```python
from build123d import *

# Parameters (mm, degrees)
F1_DEPTH = 2


with BuildPart() as f1:
    # F0 (on Top) → F1 (new body)
    with BuildSketch(Plane.XY):
        with BuildLine():
            Line((4.733724, -4.386716), (4.733724, -3.120114))
            ThreePointArc((4.733724, -3.120114), (0.208889, 1.143126), (-4.315945, -3.120114))
            Line((-4.315945, -3.120114), (-4.315945, -4.386716))
            Line((-4.315945, -4.386716), (4.733724, -4.386716))
        make_face()
        with BuildLine():
            ThreePointArc((-4.14372, -3.151427), (0.201964, 0.973099), (4.577155, -3.120114))
            Line((4.577155, -3.120114), (3.955484, -3.151427))
            Line((3.955484, -3.151427), (3.568369, -3.014677))
            Line((3.568369, -3.014677), (1.677037, -0.935318))
            Line((1.677037, -0.935318), (1.190378, -0.603505))
            Line((1.190378, -0.603505), (0.371907, 0.336631))
            Line((0.371907, 0.336631), (0.679859, -0.437599))
            Line((0.679859, -0.437599), (0.847505, -0.603505))
            Line((0.847505, -0.603505), (1.079774, -0.935318))
            Line((1.079774, -0.935318), (1.787641, -1.51046))
            Line((1.787641, -1.51046), (2.030971, -1.897575))
            Line((2.030971, -1.897575), (3.170194, -3.014677))
            Line((3.170194, -3.014677), (3.170194, -3.151427))
            Line((3.170194, -3.151427), (2.030971, -3.151427))
            Line((2.030971, -3.151427), (1.677037, -2.328931))
            Line((1.677037, -2.328931), (1.190378, -1.51046))
            Line((1.190378, -1.51046), (0.679859, -1.03181))
            Line((0.679859, -1.03181), (0.604176, -0.761511))
            Line((0.604176, -0.761511), (0.468727, -0.277765))
            Line((0.468727, -0.277765), (0.371907, -0.304874))
            Line((0.371907, -0.304874), (0.604176, -1.134406))
            Line((0.604176, -1.134406), (1.079774, -1.753789))
            Line((1.079774, -1.753789), (1.466889, -2.616502))
            Line((1.466889, -2.616502), (1.466889, -3.151427))
            Line((1.466889, -3.151427), (-0.822619, -3.151427))
            Line((-0.822619, -3.151427), (-0.822619, -3.014677))
            Line((-0.822619, -3.014677), (-0.512927, -2.793469))
            Line((-0.512927, -2.793469), (0.217061, -1.610004))
            Line((0.217061, -1.610004), (0, 0.458295))
            Line((0, 0.458295), (-0.822619, -0.304874))
            Line((-0.822619, -0.304874), (-1.618969, -1.388795))
            Line((-1.618969, -1.388795), (-1.818057, -1.388795))
            Line((-1.818057, -1.388795), (-3.233791, -3.014677))
            Line((-3.233791, -3.014677), (-3.47712, -3.014677))
            Line((-3.47712, -3.014677), (-3.654087, -3.151427))
            Line((-3.654087, -3.151427), (-4.14372, -3.151427))
        make_face(mode=Mode.SUBTRACT)
    extrude(amount=F1_DEPTH)


solid = f1.part
```
CAD build for the part. Positions are in the model's coordinates, mm. A direction names the side the tool comes from. Coordinates: 2 decimals unless noted, no trailing zeros. Write each loop counter-clockwise with the first axis right and the second up, starting at its lowest first coordinate (ties: lowest second). Pieces come first, ordered by that corner, then holes. Notation, with made-up numbers: (14, 69) -> (53, 69) arc R21 cw to (53, 79) -> close; hole circle Ø11 at (35, 17). An arc over 180 degrees is marked (long way). Use CSV: the item, a comma, the result in double quotes. Start each with the question number.
Item 1: Two-plate mould, pull along Y, no slides. Class faces 1 (the flat face through (-1, -3, 0)), 2 (the flat face through (3, -3.151, 1)), 3 (the cylindrical face through (0.305, 1.142, 0.986)), 4 (the flat face through (1.27, -2.18, 0.99)): +Y half, -Y half, draft (parallel to the pull), parting line (faces both ways), or undercut.
Item 2: Wall check: probe 1 along Y at (x, z) = (2.5, 0.2); probe 2 along X at (y, z) = (-1.9, 0.3); probe 3 along Y at (x, z) = (3, 0.3). Give the ranges that are in metal, low to high.
Item 3: Tool access for faces 5 (the flat face through (0, -4.387, 1)), 6 (the flat face through (-0.41, 0.08, 0.99)): list every direction of +Z, -Z, +X, -X, +Y, -Y with a clear straight run to the whole face (end or side of a thin tool).
Item 4: Drop a flat-ended pin along its axis: P1, Ø0.9, axis at x = 2.5, z = 1.5, coming from the +Y side. Give the stop position or say it passes through.
Item 5: Band-saw the part on D-D, the plane y = -2.5. Write the cut outline in (x, z), plus the area to 3 significant figures.
Item 6: Band-saw the part on C-C, the plane x = 2.5. Write the cut outline in (y, z), plus the area to 3 significant figures.
Item 7: Band-saw the part on B-B, the plane y = 0.8. Write the cut outline in (x, z).
Item 8: Band-saw the part on A-A, the plane x = -2. Write the cut outline in (y, z).
Response values:
1,face 1,"draft"
1,face 2,"undercut"
1,face 3,"+Y half"
1,face 4,"undercut"
2,probe 1,"y = -4.39 to -3.15, -2.36 to -1.84, 0.33 to 0.52"
2,probe 2,"x = -4.07 to -3.89, -2.26 to 0.04, 1.15 to 1.42, 2.03 to 2.55, 4.32 to 4.49"
2,probe 3,"y = -4.39 to -3.15, -2.85 to -2.39, -0.03 to 0.18"
3,face 5,"+Z, -Z, +X, -X, -Y"
3,face 6,"+Z, -Z"
4,P1,"stops at y = 0.75"
5,outline,"(-4.24, 0) -> (-4.06, 0) -> (-4.06, 2) -> (-4.24, 2) -> close; (-2.79, 0) -> (-0.33, 0) -> (-0.33, 2) -> (-2.79, 2) -> close; (1.41, 0) -> (1.75, 0) -> (1.75, 2) -> (1.41, 2) -> close; (2.65, 0) -> (3.1, 0) -> (3.1, 2) -> (2.65, 2) -> close; (4.49, 0) -> (4.65, 0) -> (4.65, 2) -> (4.49, 2) -> close"
5,area,"7.17 mm2"
6,outline,"(-4.39, 0) -> (-3.15, 0) -> (-3.15, 2) -> (-4.39, 2) -> close; (-2.36, 0) -> (-1.84, 0) -> (-1.84, 2) -> (-2.36, 2) -> close; (0.33, 0) -> (0.52, 0) -> (0.52, 2) -> (0.33, 2) -> close"
6,area,"3.89 mm2"
7,outline,"(-1.52, 0) -> (-1, 0) -> (-1, 2) -> (-1.52, 2) -> close; (1.44, 0) -> (1.94, 0) -> (1.94, 2) -> (1.44, 2) -> close"
8,outline,"(-4.39, 0) -> (-1.6, 0) -> (-1.6, 2) -> (-4.39, 2) -> close; (0.37, 0) -> (0.57, 0) -> (0.57, 2) -> (0.37, 2) -> close"
